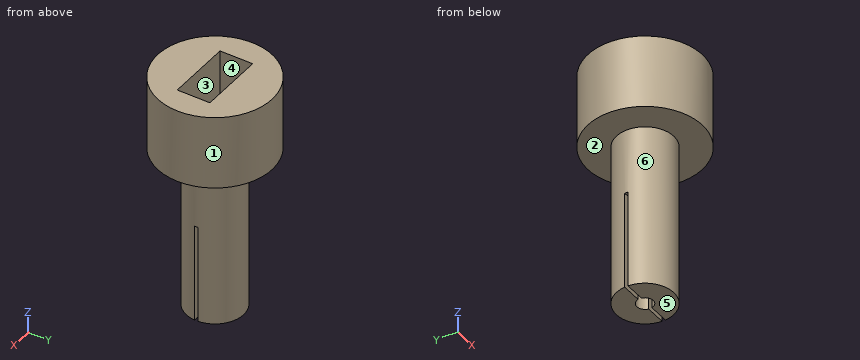
Autodesk Inventor part; units mm, degrees
ref_plane "YZ Plane" through (0, 0, 0) normal (1, 0, 0) x (0, 1, 0)
ref_plane "XZ Plane" through (0, 0, 0) normal (0, 1, 0) x (-1, 0, 0)
ref_plane "XY Plane" through (0, 0, 0) normal (0, 0, 1) x (1, 0, 0)
sketch "Sketch1" plane through (0, 0, 0) normal (0, 0, 1) x (1, 0, 0)
  circle A0 centre (0, 0) radius 1.75
  dimension "d0" = 3.5
extrude "Extrusion1" add sketch "Sketch1" along normal blind 10
sketch "Sketch2" plane through (0, 0, 10) normal (0, 0, 1) x (1, 0, 0)
  circle A0 centre (0, 0) radius 3.5
  dimension "d3" = 7
extrude "Extrusion2" add sketch "Sketch2" along normal blind 4.5
sketch "Sketch3" plane through (0, 0, 14.5) normal (0, 0, 1) x (1, 0, 0)
  line L0 (-2, 1) -> (2, 1)
  line L1 (2, 1) -> (2, -1)
  line L2 (2, -1) -> (-2, -1)
  line L3 (-2, -1) -> (-2, 1)
  point P0 (0, 0)
  point P1 (-2, 0)
  point P2 (0, 1)
  dimension "d6" = 4
  dimension "d7" = 2
extrude "Extrusion3" cut sketch "Sketch3" against normal blind 4
sketch "Sketch4" plane through (0, 0, 0) normal (0, 0, -1) x (-1, 0, 0)
  circle A0 centre (0, 0) radius 0.5
  line L0 (2, -0.1) -> (-2, -0.1)
  line L1 (-2, -0.1) -> (-2, 0.1)
  line L2 (-2, 0.1) -> (2, 0.1)
  line L3 (2, 0.1) -> (2, -0.1)
  point P0 (0, -0.1)
  point P1 (2, 0)
  point P2 (-0.4899, 0.1)
  point P3 (-0.4899, -0.1)
  point P4 (0.4899, -0.1)
  point P5 (0.4899, 0.1)
  dimension "d10" = 1
  dimension "d11" = 4
  dimension "d12" = 0.2
extrude "Extrusion4" cut sketch "Sketch4" against normal blind 6
properties part number "Magnethalter"
Verification items for the finished model (mm, model axes). Face numbers are marked on the shaded views. A direction names the side the tool comes from. Coordinates: 2 decimals unless noted, no trailing zeros. Loops run counter-clockwise (first coordinate to the right, second up) from the corner with the lowest first, then second, coordinate; pieces in that order, holes last. Notation, with made-up numbers: (72.25, 61) -> (79.25, 61) arc R28 ccw to (79.25, 84) -> close; hole circle Ø2 at (64.25, 71.25). An arc over 180 degrees is marked (long way). Put each result on its own line as item: value.
1. Gauge pin test, flat ends, axial feed: P1, Ø0.6, axis at x = -1, z = 4.5, coming from the +Y side; P2, Ø4, axis at y = -2, z = 7.5, coming from the +X side; P3, Ø1.4, axis at x = 1, z = 2, coming from the -Y side. Record the tip position at first contact, or that the pin passes through.
Result set:
P1: stops at y = 1.6
P2: stops at x = 1.75
P3: stops at y = -1.72
2. Mould release check, pull along X, two halves, no side actions. Record for the marked faces 4, 5 and 6: pulls with the +X half, pulls with the -X half, needs draft (parallel to the pull), parting line crosses it, or undercut.
Result set:
face 4: undercut
face 5: needs draft
face 6: parting line crosses it
3. Section check A-A, the plane x = 0. Record the boundary of the cut face in (y, z), then the cut area to 3 significant figures.
Result set:
outline: (-3.5, 10) -> (-1.75, 10) -> (-1.75, 0) -> (-0.5, 0) -> (-0.5, 6) -> (0.5, 6) -> (0.5, 0) -> (1.75, 0) -> (1.75, 10) -> (3.5, 10) -> (3.5, 14.5) -> (1, 14.5) -> (1, 10.5) -> (-1, 10.5) -> (-1, 14.5) -> (-3.5, 14.5) -> close
area: 52.5 mm^2
4. Thickness scan on line 1 (Y direction, x = 1.25, z = 1); line 2 (X direction, y = -0.25, z = 13.25); line 3 (Z direction, x = -1, y = 2.5). Record the ranges inside material, lowest first.
Result set:
line 1: y = -1.22 to -0.1, 0.1 to 1.22
line 2: x = -3.49 to -2, 2 to 3.49
line 3: z = 10 to 14.5
5. Section check D-D, the plane y = 2. Record the boundary of the cut face in (x, z), then the cut area to 3 significant figures.
Result set:
outline: (-2.87, 10) -> (2.87, 10) -> (2.87, 14.5) -> (-2.87, 14.5) -> close
area: 25.9 mm^2
6. Section check C-C, the plane y = 2.75. Record the boundary of the cut face in (x, z).
Result set:
outline: (-2.17, 10) -> (2.17, 10) -> (2.17, 14.5) -> (-2.17, 14.5) -> close
7. Tool access check on the marked faces 1, 2 and 3. Record the directions out of +Z, -Z, +X, -X, +Y, -Y that give a thin tool (end or side, any length) a straight path to the whole face; none if there is none.
Result set:
face 1: +Z, -Z
face 2: -Z
face 3: +Z
8. Section check B-B, the plane y = 0.25. Record the boundary of the cut face in (x, z).
Result set:
outline: (-3.49, 10) -> (-1.73, 10) -> (-1.73, 0) -> (-0.43, 0) -> (-0.43, 6) -> (0.43, 6) -> (0.43, 0) -> (1.73, 0) -> (1.73, 10) -> (3.49, 10) -> (3.49, 14.5) -> (2, 14.5) -> (2, 10.5) -> (-2, 10.5) -> (-2, 14.5) -> (-3.49, 14.5) -> close
